```python
from build123d import *

# Parameters (mm, degrees)
BOSS_EXTRUDE1_DEPTH     = 10
FILLET1_R               = 10
CUT_EXTRUDE1_DEPTH      = 59.446556785
CUT_EXTRUDE1_DEPTH_BACK = 59.446556785
SKETCH3_R               = 1.625
FILLET2_R               = 10
SKETCH4_R               = 2.5
CUT_EXTRUDE2_DEPTH      = 55.772255751
SKETCH5_W               = 20
SKETCH5_H               = 12
CUT_EXTRUDE3_DEPTH      = 59.446556785
FILLET3_R               = 10
FILLET5_R               = 0.5
FILLET6_R               = 2


with BuildPart() as part:
    # Sketch1 → Boss-Extrude1 (new, symmetric)
    with BuildSketch(Plane.XY):
        Polygon((0, 0), (0, -20), (-4, -20), (-4, -7), (-54, -7), (-54, -4), (-34, -4), (-34, -3), (-54, -3), (-54, 0), align=None)
    extrude(amount=BOSS_EXTRUDE1_DEPTH, both=True)

    # Fillet1
    fillet1_edges = [part.edges().sort_by_distance(p)[0] for p in [
        (-54, -5.5, -10),
        (-54, -1.5, -10),
        (-54, -5.5, 10),
        (-54, -1.5, 10),
    ]]
    fillet(fillet1_edges, radius=FILLET1_R - 0.0001)  # a hair under: the kernel refuses the full size

    # Sketch3 → Cut-Extrude1 (cut, two sides: drawn at the far end of the back side and taken through both)
    with BuildSketch(Plane(origin=(0, 0, 0), x_dir=(1, 0, 0), z_dir=(0, 1, 0)).offset(-CUT_EXTRUDE1_DEPTH_BACK)):
        with Locations(Location((-51.071067812, 0, 0), (0, 0, 180))):
            Circle(SKETCH3_R)
        with Locations(Location((-41.071067812, 0, 0), (0, 0, 180))):
            Circle(SKETCH3_R)
        with Locations(Location((-31.071067812, 0, 0), (0, 0, 180))):
            Circle(SKETCH3_R)
    extrude(amount=CUT_EXTRUDE1_DEPTH + CUT_EXTRUDE1_DEPTH_BACK, mode=Mode.SUBTRACT)

    # Fillet2
    fillet2_edges = [part.edges().sort_by_distance(p)[0] for p in [
        (-2, -20, 10),
        (-2, -20, -10),
    ]]
    fillet(fillet2_edges, radius=FILLET2_R - 0.0001)  # a hair under: the kernel refuses the full size

    # Sketch4 → Cut-Extrude2 (cut, through all)
    with BuildSketch(Plane.ZY.offset(4)):
        with Locations((0, -13)):
            Circle(SKETCH4_R)
    extrude(amount=-CUT_EXTRUDE2_DEPTH, mode=Mode.SUBTRACT)

    # Sketch5 → Cut-Extrude3 (cut, through all)
    with BuildSketch(Plane(origin=(0, 0, 0), x_dir=(1, 0, 0), z_dir=(0, 1, 0))):
        with Locations((-14, 0)):
            Rectangle(SKETCH5_W, SKETCH5_H)
    extrude(amount=-CUT_EXTRUDE3_DEPTH, mode=Mode.SUBTRACT)

    # Fillet3
    fillet3_edges = [part.edges().sort_by_distance(p)[0] for p in [
        (-4, -7, -8),
        (-4, -7, 8),
    ]]
    fillet(fillet3_edges, radius=FILLET3_R)

    # Fillet5
    fillet5_edges = [part.edges().sort_by_distance(p)[0] for p in [
        (-4, -19.219544127, -3.873063981),
        (-4.63248147, -13.50005763, -9.367506076),
        (-10.126952105, -7.780482659, -10),
        (-10.126952105, -7.780482659, 10),
        (-4.63248147, -13.50005763, 9.367506076),
        (-39.00005, -4, -10),
        (-22.00005, 0, -10),
        (-34, -3.5, 10),
        (-39.00005, -4, 10),
        (-29.00005, -7, -10),
        (-29.00005, -7, 10),
        (-51.071097101, -7, 7.071097101),
        (-51.071097101, -7, -7.071097101),
        (-39.00005, -3, -10),
        (-51.071097101, -4, 7.071097101),
        (-51.071097101, -4, -7.071097101),
        (-39.00005, -3, 10),
        (-51.071097101, -3, 7.071097101),
        (-51.071097101, -3, -7.071097101),
        (-51.071097101, 0, 7.071097101),
        (-51.071097101, 0, -7.071097101),
        (-22.00005, 0, 10),
        (0, -5.00005, 10),
        (0, -5.00005, -10),
        (0, -17.071097101, -7.071097101),
        (0, -17.071097101, 7.071097101),
        (-4, -19.219544127, 3.873063981),
    ]]
    fillet(fillet5_edges, radius=FILLET5_R)

    # Fillet6
    fillet6_edges = [part.edges().sort_by_distance(p)[0] for p in [
        (-24, -3.5, 6),
        (-4, -8.5, 6),
        (-24, -3.5, -6),
        (-4, -8.5, -6),
    ]]
    fillet(fillet6_edges, radius=FILLET6_R)


solid = part.part
```
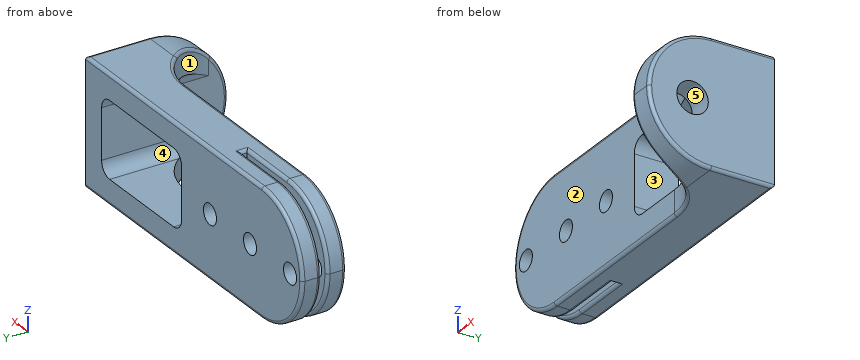
Work out the finished part from the listing and answer in its coordinate system (mm). Face numbers are marked on the shaded views. A direction names the side the tool comes from. Round coordinates to 2 decimals unless told otherwise and drop trailing zeros. Loops run counter-clockwise (first coordinate to the right, second up) from the corner with the lowest first, then second, coordinate; pieces in that order, holes last. Notation, with made-up numbers: M 61.25,6 L 114.25,6 A22 cw 114.25,32 Z; hole C -6,37.25 d4. An arc over 180 degrees is marked long. Use CSV: the item, a comma, the result in double quotes.
Q1. Section A-A, the plane x = -28 is taken. Determine the outline of the cut face in (y, z).
Determined:
outline,"M -7,-9.5 A0.5 ccw -6.5,-10 L -0.5,-10 A0.5 ccw 0,-9.5 L 0,9.5 A0.5 ccw -0.5,10 L -6.5,10 A0.5 ccw -7,9.5 Z"
Q2. The mould has two halves that part along X. Classify the marked faces 1, 2 and 3: pulls with the +X half, pulls with the -X half, needs draft (parallel to the pull), parting line crosses it, or undercut.
Determined:
face 1,"pulls with the -X half"
face 2,"needs draft"
face 3,"undercut"
Q3. Section B-B, the plane z = -0.75 is taken. State how many separate pieces and enclosed holes the cut face has, then the cut area to 3 significant figures.
Determined:
separate pieces,"8"
enclosed holes,"0"
area,"196 mm2"
Q4. A tool of negligible diameter and unlimited length cuts with its end or side. For the marked faces 4 and 5, from which of +Z, -Z, +X, -X, +Y, -Y can it reach the whole face along a straight path? Write none if from no direction.
Determined:
face 4,"+Y, -Y"
face 5,"+X, -X"
Q5. Each of these flat-tipped pins is pushed along its axis until it touches: pin 1 (3.5 mm diameter, centred on x = -51.07, z = 0, fed in from -Y); pin 2 (6.5 mm diameter, centred on y = -12, z = -2.5, fed in from -X); pin 3 (0.6 mm diameter, centred on y = -3, z = -3, fed in from -X); pin 4 (1.9 mm diameter, centred on x = -31.07, z = 0, fed in from +Y). Where does it stop, or does it pass through?
Determined:
pin 1,"y = -7"
pin 2,"x = -5.03"
pin 3,"x = -53.52"
pin 4,"through"
Q6. Consider L1, parallel to X at y = -5.4, z = 0; L2, parallel to Y at x = -2.2, z = 0; L3, parallel to Y at x = -43, z = -6.5. Determine where each line is inside the solid, lowest interval first.
Determined:
L1,"-54 to -52.7, -49.45 to -42.7, -39.45 to -32.7, -29.45 to -24, -4 to 0"
L2,"-20 to -15.5, -10.5 to 0"
L3,"-7 to -4, -3 to 0"
